```python
from build123d import *

# Parameters (mm, degrees)
SKETCH1_R           = 1.6
BOSS_EXTRUDE1_DEPTH = 100
SKETCH2_W           = 8.75
SKETCH2_H           = 20
CUT_EXTRUDE1_DEPTH  = 100
SKETCH3_W           = 25
SKETCH3_H           = 20
BOSS_EXTRUDE2_DEPTH = 60
SKETCH4_R           = 1.25
CUT_EXTRUDE2_DEPTH  = 60
CHAMFER1_SIZE       = 3


with BuildPart() as part:
    # Sketch1 → Boss-Extrude1 (new body)
    with BuildSketch(Plane(origin=(0, 0, 0), x_dir=(1, 0, 0), z_dir=(0, 1, 0))):
        Polygon((-17.25, -10), (17.25, -10), (25.25, -10), (25.25, 10), (17.25, 10), (-17.25, 10), align=None)
        with Locations(Location((-5, 5, 0), (0, 0, 270))):
            Circle(SKETCH1_R, mode=Mode.SUBTRACT)
        with Locations(Location((13, 5, 0), (0, 0, 270))):
            Circle(SKETCH1_R, mode=Mode.SUBTRACT)
        with Locations(Location((-5, -5, 0), (0, 0, 270))):
            Circle(SKETCH1_R, mode=Mode.SUBTRACT)
        with Locations(Location((13, -5, 0), (0, 0, 270))):
            Circle(SKETCH1_R, mode=Mode.SUBTRACT)
    extrude(amount=BOSS_EXTRUDE1_DEPTH)

    # Sketch2 → Cut-Extrude1 (cut)
    with BuildSketch(Plane.XZ):
        with Locations((-12.875, 0)):
            Rectangle(SKETCH2_W, SKETCH2_H)
        with Locations((20.875, 0)):
            Rectangle(SKETCH2_W, SKETCH2_H)
    extrude(amount=-CUT_EXTRUDE1_DEPTH, mode=Mode.SUBTRACT)

    # Sketch3 → Boss-Extrude2 (add)
    with BuildSketch(Plane(origin=(0, 100, 0), x_dir=(1, 0, 0), z_dir=(0, 1, 0))):
        with Locations((4, 0)):
            Rectangle(SKETCH3_W, SKETCH3_H)
    extrude(amount=-BOSS_EXTRUDE2_DEPTH)

    # Sketch4 → Cut-Extrude2 (cut)
    with BuildSketch(Plane.XY.offset(10)):
        with Locations((4, 50)):
            Circle(SKETCH4_R)
        with Locations((4, 70)):
            Circle(SKETCH4_R)
        with Locations((4, 90)):
            Circle(SKETCH4_R)
    extrude(amount=-CUT_EXTRUDE2_DEPTH, mode=Mode.SUBTRACT)

    # Chamfer1
    chamfer1_edges = [part.edges().sort_by_distance(p)[0] for p in [
        (4, 0, 10),
        (4, 100, 10),
        (-8.5, 50, 10),
        (16.5, 50, 10),
    ]]
    chamfer(chamfer1_edges, length=CHAMFER1_SIZE)


solid = part.part
```
Design review of the part built by this model. Coordinates are the model's own, in mm. A direction names the side the tool comes from. Coordinates: 2 decimals unless noted, no trailing zeros. Order: outer loops, then holes, each group sorted by start corner. A loop starts at its lowest first (then second) coordinate and runs counter-clockwise, first axis right, second up. Notation, with made-up numbers: (3.5, 58.25) -> (29.5, 58.25) arc R24 cw to (29.5, 74.25) -> close; hole circle Ø4 at (31, 37). An arc over 180 degrees is marked (long way). One line per item, written item: value. Start each with the question number.
Q1. Take a section at C-C, the plane z = 5. State the section outline as (x, y) points, then the cut area to 3 significant figures.
Q2. Take a section at A-A, the plane x = 4. State the section outline as (y, z) points, then the cut area to 3 significant figures.
Q3. Mouldability with a two-part tool opening along Z and no side actions: class faces 1 (the cylindrical face through (-4.519, 19.72, 6.526)), 2 (the flat face through (4, 99, 8)), 3 (the cylindrical face through (3.84, 51.24, 0.14)) as pulls with the +Z half, pulls with the -Z half, needs draft (parallel to the pull), parting line crosses it, or undercut.
Q4. Take a section at B-B, the plane y = 90. State the section outline as (x, z) points.
Q5. For probe 1 along Z at (x, y) = (13, 27.5); probe 2 along Y at (x, z) = (4, -1.5); probe 3 along X at (y, z) = (17.5, 5), list the stretches that pass through material, from the lowest coordinate up.
Q6. Tool access review of faces 4 (the flat face through (-7, 50.7, 8.5)), 5 (the flat face through (-5, 40, -5)): name each direction out of +Z, -Z, +X, -X, +Y, -Y from which nothing blocks a thin tool from reaching the whole face with its end or side.
Q7. Take a section at D-D, the plane y = 6. State the section outline as (x, z) points.
Q8. Insertion check: pin 1 Ø2 at (x, y) = (4, 90) entering from -Z; pin 2 Ø10 at (x, z) = (2.5, -2.5) entering from -Y; pin 3 Ø1 at (x, z) = (-4, -5) entering from -Y. Each pin has a flat end and moves straight along its axis. Give the tip position at first contact, or say it passes through.
Values follow:
1. outline: (-8.5, 0) -> (-6.6, 0) -> (-6.6, 40) -> (-3.4, 40) -> (-3.4, 0) -> (11.4, 0) -> (11.4, 40) -> (14.6, 40) -> (14.6, 0) -> (16.5, 0) -> (16.5, 100) -> (-8.5, 100) -> close; hole circle Ø2.5 at (4, 50); hole circle Ø2.5 at (4, 70); hole circle Ø2.5 at (4, 90)
1. area: 2,230 mm2
2. outline: (0, -10) -> (48.75, -10) -> (48.75, 10) -> (3, 10) -> (0, 7) -> close; (51.25, -10) -> (68.75, -10) -> (68.75, 10) -> (51.25, 10) -> close; (71.25, -10) -> (88.75, -10) -> (88.75, 10) -> (71.25, 10) -> close; (91.25, -10) -> (100, -10) -> (100, 7) -> (97, 10) -> (91.25, 10) -> close
2. area: 1,840 mm2
3. face 1: undercut
3. face 2: pulls with the +Z half
3. face 3: needs draft
4. outline: (-8.5, -10) -> (2.75, -10) -> (2.75, 10) -> (-5.5, 10) -> (-8.5, 7) -> close; (5.25, -10) -> (16.5, -10) -> (16.5, 7) -> (13.5, 10) -> (5.25, 10) -> close
5. probe 1: z = -10 to -6.6, -3.4 to 3.4, 6.6 to 10
5. probe 2: y = 0 to 48.75, 51.25 to 68.75, 71.25 to 88.75, 91.25 to 100
5. probe 3: x = -8.5 to -6.6, -3.4 to 11.4, 14.6 to 16.5
6. face 4: +Z, -X, +Y, -Y
6. face 5: -Y
7. outline: (-8.5, -10) -> (16.5, -10) -> (16.5, 7) -> (13.5, 10) -> (-5.5, 10) -> (-8.5, 7) -> close; hole circle Ø3.2 at (-5, -5); hole circle Ø3.2 at (-5, 5); hole circle Ø3.2 at (13, -5); hole circle Ø3.2 at (13, 5)
8. pin 1: passes through
8. pin 2: stops at y = 0
8. pin 3: stops at y = 40
